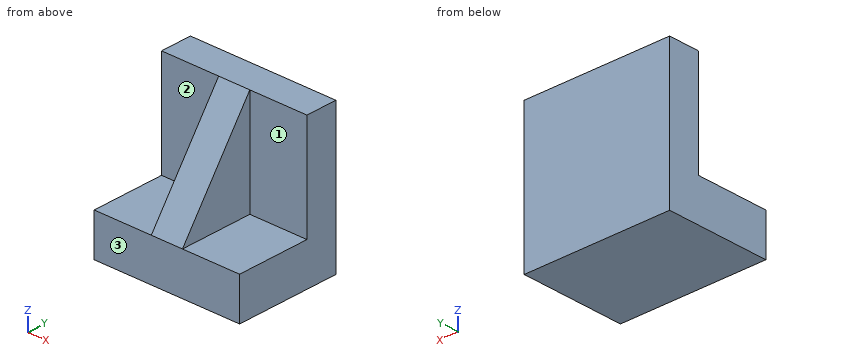
```python
from build123d import *

# Parameters (mm, degrees)
F0_W     = 70
F0_H     = 35
F1_DEPTH = 20
F0_H_2   = 15
F2_DEPTH = 70
F4_DEPTH = 7.5


with BuildPart() as f1:
    # F0 (on Top) → F1 (new body)
    with BuildSketch(Plane.XY):
        with Locations((0, -42.5)):
            Rectangle(F0_W, F0_H)
    extrude(amount=F1_DEPTH)

    # F0 (on Top) → F2 (join)
    with BuildSketch(Plane.XY):
        with Locations((0, -17.5)):
            Rectangle(F0_W, F0_H_2)
    extrude(amount=F2_DEPTH)

    # F3 (on Right) → F4 (join, symmetric)
    with BuildSketch(Plane.YZ):
        Polygon((-25, 20), (-25, 70), (-60, 20), align=None)
    extrude(amount=F4_DEPTH, both=True)


solid = f1.part
```
Part model, mm, in its own coordinate system. Face numbers are marked on the shaded views. A direction names the side the tool comes from. Coordinates: 2 decimals unless noted, no trailing zeros. Loops run counter-clockwise (first coordinate to the right, second up) from the corner with the lowest first, then second, coordinate; pieces in that order, holes last. Notation, with made-up numbers: (-16, -25.75) - (1, -25.75) arc R16 cw to (1, -15.75) - close; hole circle Ø11 at (67.5, -25.5). An arc over 180 degrees is marked (long way). Write item = value, one per line. Start each with the question number.
Item 1: 3-axis set-ups, long thin cutter, end or side, ignore diameter. For the marked faces 1, 2 and 3: which of +Z, -Z, +X, -X, +Y, -Y reach the whole face in a straight line?
Item 2: Flat gauge pins, fed straight in: pin 1 Ø10.5 at (y, z) = (-43.5, 32.5) entering from +X; pin 2 Ø22 at (x, y) = (-25, -45) entering from +Z; pin 3 Ø17.5 at (y, z) = (-43.5, 52) entering from -X. Where does each tip first touch, or does it go through?
Item 3: Cut at B-B, the plane y = -54. Give the cut face in (x, z).
Item 4: Cut at C-C, the plane x = 22.5. Give the cut face in (y, z), and give its area (3 significant figures).
Item 5: Cut at A-A, the plane z = 25.5. Give the cut face in (x, y).
Item 6: Cut at D-D, the plane x = 5. Give the cut face in (y, z), and give its area (4 significant figures).
Item 7: Wall check: L1, parallel to Z at x = -26, y = -33.5; L2, parallel to Y at x = -26, z = 55; L3, parallel to X at y = -31, z = 35. Give the ranges that are in metal, low to high. Write a range as from..to.
The answers:
q1.face_1 = +Z, +X, -Y
q1.face_2 = +Z, -X, -Y
q1.face_3 = +Z, -Z, +X, -X, -Y
q2.pin_1 = 7.5
q2.pin_2 = 20
q2.pin_3 = -7.5
q3.outline = (-35, 0) - (35, 0) - (35, 20) - (7.5, 20) - (7.5, 28.57) - (-7.5, 28.57) - (-7.5, 20) - (-35, 20) - close
q4.outline = (-60, 0) - (-10, 0) - (-10, 70) - (-25, 70) - (-25, 20) - (-60, 20) - close
q4.area = 1,750 mm2
q5.outline = (-35, -25) - (-7.5, -25) - (-7.5, -56.15) - (7.5, -56.15) - (7.5, -25) - (35, -25) - (35, -10) - (-35, -10) - close
q6.outline = (-60, 0) - (-10, 0) - (-10, 70) - (-25, 70) - (-60, 20) - close
q6.area = 2,625 mm2
q7.L1 = 0..20
q7.L2 = -25..-10
q7.L3 = -7.5..7.5
